Geometry check sheet. Reference: the model listing, model coordinates, mm. Round coordinates to 2 decimals unless told otherwise and drop trailing zeros. Write each loop counter-clockwise with the first axis right and the second up, starting at its lowest first coordinate (ties: lowest second). Pieces come first, ordered by that corner, then holes.
from build123d import *

# Parameters (mm, degrees)
PAD006_DEPTH    = 10
SKETCH008_R     = 2.106519
POCKET001_DEPTH = 10.001
SKETCH013_R     = 3
POCKET003_DEPTH = 10.001


with BuildPart() as part:
    # Sketch007 → Pad006 (new body)
    with BuildSketch(Plane.XZ.offset(67)):
        with BuildLine():
            Line((-44.627205, 4.223839), (-5.639042, 4.223839))
            Line((-5.639042, 4.223839), (-5.639042, -17.503959))
            ThreePointArc((-25.234732, -37.099649), (-11.378487, -31.360204), (-5.639042, -17.503959))
            Line((-25.234732, -37.099649), (-44.627205, -37.099649))
            Line((-44.627205, -37.099649), (-44.627205, 4.223839))
        make_face()
    extrude(amount=PAD006_DEPTH)

    # Sketch008 (on Face6 of Pad006) → Pocket001 (cut, through all)
    with BuildSketch(Plane(origin=(0, -67, 1), x_dir=(1, 0, 0), z_dir=(0, 1, 0))):
        with Locations((-24.808006, 0.705665)):
            Circle(SKETCH008_R)
    extrude(amount=-POCKET001_DEPTH, mode=Mode.SUBTRACT)

    # Sketch013 (on Face5 of Pocket001) → Pocket003 (cut, through all)
    with BuildSketch(Plane.XZ.offset(77)):
        with Locations((-25.001532, -18.014723)):
            Circle(SKETCH013_R)
    extrude(amount=-POCKET003_DEPTH, mode=Mode.SUBTRACT)


with BuildPart() as part_1:
    # Body004 placement: moved
    add(part.part.moved(Location((0, 0, 7))))


solid = part_1.part
1. Scan lines: line 1 along X through (y, z) = (-71, -28); line 2 along Z through (x, y) = (-11.5, -67.25); line 3 along X through (y, z) = (-76, -21). Record each from-to range of solid material in increasing order.
2. Section check C-C (z = -20.5). Record the cut outline in (x, y).
3. Section check D-D (x = -11.5). Record the cut outline in (y, z), plus the area to 3 significant figures.
4. Release check for a two-part mould opening along Z. For faces 1 (the face through (-29, -77, -9)), 2 (the face through (-22.8, -71.93, 6.66)), 3 (the face through (-11.53, -71.93, -24.51)) record: +Z half, -Z half, draft (parallel to the pull), parting line (faces both ways), or undercut.
5. Depth check by flat-ended pin: pin 1 Ø3 at (y, z) = (-74, -13) entering from +X. Enter the tip coordinate at first touch or a pass-through.
6. Section check B-B (y = -72.5). Record the cut outline in (x, z).
7. Section check A-A (x = -26). Record the cut outline in (y, z), plus the area to 3 significant figures.
Results below:
1. line 1: x = -44.63 to -16.41
1. line 2: z = -24.48 to 11.22
1. line 3: x = -44.63 to -8.69
2. outline: (-44.63, -77) - (-8.38, -77) - (-8.38, -67) - (-44.63, -67) - close
3. outline: (-77, -24.48) - (-67, -24.48) - (-67, 11.22) - (-77, 11.22) - close
3. area: 357 mm2
4. face 1: draft
4. face 2: undercut
4. face 3: -Z half
5. pin 1: stops at x = -5.66
6. outline: (-44.63, -30.1) - (-25.23, -30.1) arc R19.6 ccw to (-5.64, -10.5) - (-5.64, 11.22) - (-44.63, 11.22) - close; hole circle Ø6 at (-25, -11.01); hole circle Ø4.21 at (-24.81, 7.29)
7. outline: (-77, -30.1) - (-67, -30.1) - (-67, -13.84) - (-77, -13.84) - close; (-77, -8.19) - (-67, -8.19) - (-67, 5.56) - (-77, 5.56) - close; (-77, 9.03) - (-67, 9.03) - (-67, 11.22) - (-77, 11.22) - close
7. area: 322 mm2
